from build123d import *

# Parameters (mm, degrees)
F0_W        = 45
F0_H        = 5
F1_DEPTH    = 40
F2_T1_DEPTH = 40
F2_T3_DEPTH = 65
F2_T5_DEPTH = 54.4889687993
F2_T7_DEPTH = 46.9752871377
F3_R        = 39.6889865909


# Not quite as in the source:
# - a fillet or chamfer that OpenCascade refuses, or shapes differently, is made with other operations: its cross-section is extruded or revolved along the edge and cut away or added


with BuildPart() as f1:
    # F0 (on Top) → F1 (new body)
    with BuildSketch(Plane.XY):
        with Locations((27.5, 13.2681977808)):
            Rectangle(F0_W, F0_H)
        with BuildLine():
            Line((50, 10.7681977808), (50, -3.9824241135))
            ThreePointArc((50, -3.9824241135), (52.5291420669, -5.0643561015), (55, -6.273486986))
            Line((55, -6.273486986), (55, 15.7681977808))
            Line((55, 15.7681977808), (50, 15.7681977808))
            Line((50, 15.7681977808), (50, 10.7681977808))
        make_face()
        with BuildLine():
            ThreePointArc((55, -6.273486986), (52.5291420669, -5.0643561015), (50, -3.9824241135))
            Line((50, -3.9824241135), (50, -9.2318022192))
            Line((50, -9.2318022192), (50, -11.5117834926))
            ThreePointArc((50, -11.5117834926), (52.5410653135, -12.7963056669), (55, -14.2318022192))
            Line((55, -14.2318022192), (55, -6.273486986))
        make_face()
        with BuildLine():
            Line((15.8578643763, -9.2318022192), (5, -9.2318022192))
            Line((5, -9.2318022192), (5, -14.2318022192))
            ThreePointArc((5, -14.2318022192), (10.2699038194, -11.3864605272), (15.8578643763, -9.2318022192))
        make_face()
        with BuildLine():
            Line((5, -14.2318022192), (5, -9.2318022192))
            Line((5, -9.2318022192), (0, -9.2318022192))
            ThreePointArc((0, -9.2318022192), (-15, -84.2318022192), (60, -99.2318022192))
            Line((60, -99.2318022192), (60, -94.2318022192))
            Line((60, -94.2318022192), (55, -94.2318022192))
            ThreePointArc((55, -94.2318022192), (-10, -79.2318022192), (5, -14.2318022192))
        make_face()
        with BuildLine():
            ThreePointArc((15.8578643763, -9.2318022192), (10.2699038194, -11.3864605272), (5, -14.2318022192))
            Line((5, -14.2318022192), (50, -14.2318022192))
            Line((50, -14.2318022192), (50, -11.5117834926))
            ThreePointArc((50, -11.5117834926), (47.1090892478, -10.2741059066), (44.1421356237, -9.2318022192))
            Line((44.1421356237, -9.2318022192), (15.8578643763, -9.2318022192))
        make_face()
        with BuildLine():
            Line((50, -9.2318022192), (44.1421356237, -9.2318022192))
            ThreePointArc((44.1421356237, -9.2318022192), (47.1090892478, -10.2741059066), (50, -11.5117834926))
            Line((50, -11.5117834926), (50, -9.2318022192))
        make_face()
        with BuildLine():
            Line((50, -11.5117834926), (50, -14.2318022192))
            Line((50, -14.2318022192), (55, -14.2318022192))
            ThreePointArc((55, -14.2318022192), (52.5410653135, -12.7963056669), (50, -11.5117834926))
        make_face()
    extrude(amount=F1_DEPTH)

    # F2: fillet of radius 5 on 8 edges, made by hand

    # F2_s2 → F2_t1 (join)
    with BuildSketch(Plane.XY):
        with BuildLine():
            ThreePointArc((50, -4.2318022192), (48.5355339059, -7.7673361251), (45, -9.2318022192))
            Line((45, -9.2318022192), (50, -9.2318022192))
            Line((50, -9.2318022192), (50, -4.2318022192))
        make_face()
        with BuildLine():
            ThreePointArc((45, 10.7681977808), (48.5355339059, 9.3037316868), (50, 5.7681977808))
            Line((50, 5.7681977808), (50, 10.7681977808))
            Line((50, 10.7681977808), (45, 10.7681977808))
        make_face()
    extrude(amount=F2_T1_DEPTH)

    # F2_s4 → F2_t3 (cut)
    with BuildSketch(Plane.XY.offset(-12.5)):
        with BuildLine():
            ThreePointArc((55, -9.2318022192), (53.5355339059, -12.7673361251), (50, -14.2318022192))
            Line((50, -14.2318022192), (55, -14.2318022192))
            Line((55, -14.2318022192), (55, -9.2318022192))
        make_face()
        with BuildLine():
            ThreePointArc((50, 15.7681977808), (53.5355339059, 14.3037316868), (55, 10.7681977808))
            Line((55, 10.7681977808), (55, 15.7681977808))
            Line((55, 15.7681977808), (50, 15.7681977808))
        make_face()
        with BuildLine():
            ThreePointArc((5, 10.7681977808), (6.4644660941, 14.3037316868), (10, 15.7681977808))
            Line((10, 15.7681977808), (5, 15.7681977808))
            Line((5, 15.7681977808), (5, 10.7681977808))
        make_face()
        with BuildLine():
            ThreePointArc((60, -99.2318022192), (58.5355339059, -95.6962683132), (55, -94.2318022192))
            Line((55, -94.2318022192), (60, -94.2318022192))
            Line((60, -94.2318022192), (60, -99.2318022192))
        make_face()
    extrude(amount=F2_T3_DEPTH, mode=Mode.SUBTRACT)

    # F2_s6 → F2_t5 (cut)
    with BuildSketch(Plane.XY.offset(-7.2444843997)):
        with BuildLine():
            ThreePointArc((57.546692635, -100.7740381439), (59.3435851077, -98.9477505529), (60, -96.4712069105))
            Line((60, -96.4712069105), (60, -99.2318022192))
            ThreePointArc((60, -99.2318022192), (58.7836773401, -100.019354226), (57.546692635, -100.7740381439))
        make_face()
    extrude(amount=F2_T5_DEPTH, mode=Mode.SUBTRACT)

    # F2_s8 → F2_t7 (cut)
    with BuildSketch(Plane.XY.offset(-3.4876435688)):
        with BuildLine():
            ThreePointArc((56.3950574275, -94.2318022192), (55.0843622501, -94.4066516358), (53.8653367875, -94.9189709584))
            ThreePointArc((53.8653367875, -94.9189709584), (54.4350841017, -94.5793754416), (55, -94.2318022192))
            Line((55, -94.2318022192), (56.3950574275, -94.2318022192))
        make_face()
    extrude(amount=F2_T7_DEPTH, mode=Mode.SUBTRACT)

    # F3
    f3_edges = [f1.edges().sort_by_distance(p)[0] for p in [
        (0, -9.231802, 20),
        (5, -14.231802, 20),
    ]]
    fillet(f3_edges, radius=F3_R)


solid = f1.part
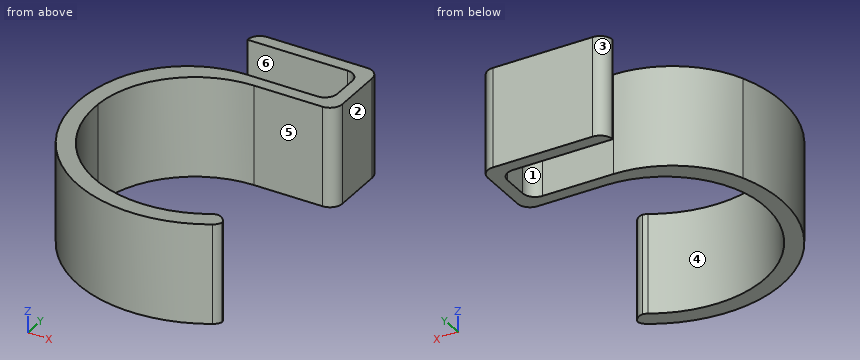
Design review of the part built by this model. Coordinates are the model's own, in mm. Face numbers are marked on the shaded views. A direction names the side the tool comes from. Round coordinates to 2 decimals unless told otherwise and drop trailing zeros. Write each loop counter-clockwise with the first axis right and the second up, starting at its lowest first coordinate (ties: lowest second). Pieces come first, ordered by that corner, then holes.
Item 1: For pin 1 Ø11 at (y, z) = (1, 20) entering from -X; pin 2 Ø12 at (x, z) = (0.5, 28) entering from +Y; pin 3 Ø20 at (x, z) = (27.5, 27) entering from -Y; pin 4 Ø12 at (y, z) = (-81.5, 29) entering from -X, all flat-tipped, find the tip position at first contact; note any pin that passes through.
Item 2: Consider section A-A on x = 24. Give the boundary of the cut face in (y, z), and give its area (3 significant figures).
Item 3: Consider section B-B on x = -0.5. Give the boundary of the cut face in (y, z).
Item 4: Consider section D-D on y = 3.5. Give the boundary of the cut face in (x, z).
Item 5: Draft analysis for pull direction Y (two halves, no side actions). For the marked faces 1, 2 and 3, state which applies: released by +Y, released by -Y, zero draft, split by the parting line, or undercut.
Item 6: Wall thickness on L1, parallel to Y at x = 18, z = 15; L2, parallel to Y at x = 33.5, z = 14.5; L3, parallel to Y at x = 51, z = 26: over which ranges is each line inside the solid? List them lowest first.
Item 7: For the marked faces 4, 5 and 6, list the 3-axis set-ups (+Z, -Z, +X, -X, +Y, -Y) from which the entire face can be reached by the end or side of a thin tool; tool diameter is ignored.
Item 8: Consider section C-C on z = 7. Give the boundary of the cut face in (x, y).
Check values:
1. pin 1: stops at x = 49.95
1. pin 2: stops at y = 14.34
1. pin 3: stops at y = -108.32
1. pin 4: stops at x = -19.73
2. outline: (-107.98, 0) - (-101.02, 0) - (-101.02, 40) - (-107.98, 40) - close; (-14.23, 0) - (-9.23, 0) - (-9.23, 40) - (-14.23, 40) - close; (10.77, 0) - (15.77, 0) - (15.77, 40) - (10.77, 40) - close
2. area: 679 mm2
3. outline: (-98.89, 0) - (-90.21, 0) - (-90.21, 40) - (-98.89, 40) - close; (-21.59, 0) - (-13.11, 0) - (-13.11, 40) - (-21.59, 40) - close
4. outline: (50, 0) - (55, 0) - (55, 40) - (50, 40) - close
5. face 1: undercut
5. face 2: zero draft
5. face 3: released by +Y
6. L1: y = -106.97 to -99.85, -14.49 to -9.23, 10.77 to 15.77
6. L2: y = -108.2 to -101.27, -14.23 to -9.23, 10.77 to 15.77
6. L3: y = -104.07 to -96.47, -14.13 to 15.67
7. face 4: +Z, -Z
7. face 5: +Z, -Z, +X
7. face 6: +Z, -Z, -X
8. outline: (-20.27, -34.28) arc R54.08 ccw to (57.55, -100.77) arc R5 ccw to (59.81, -97.85) arc R5 ccw to (55.7, -94.28) arc R5 ccw to (53.87, -94.92) arc R47.17 cw to (-17.13, -52.27) arc R39.69 cw to (22.53, -14.23) - (50, -14.23) arc R5 ccw to (55, -9.23) - (55, 10.77) arc R5 ccw to (50, 15.77) - (10, 15.77) arc R5 ccw to (5, 10.77) - (45, 10.77) arc R5 cw to (50, 5.77) - (50, -4.23) arc R5 cw to (45, -9.23) - (16.62, -9.23) arc R39.69 ccw to start
